Source: three-view drawing plus pictorial views. Frame: mm from the lowest corner of the part. A direction names the side the tool comes from. Give positions to 0.01 mm unless a question says otherwise; leave off trailing zeros. Write each loop counter-clockwise with the first axis right and the second up, starting at its lowest first coordinate (ties: lowest second). Pieces come first, ordered by that corner, then holes.
Q1. Line query: L1, parallel to Y at x = 5.9, z = 7.75; L2, parallel to Y at x = 5, z = 9.75; L3, parallel to Z at x = 1.5, y = 10.25. Output: solid intervals per line, ascending.
Q2. Cut plane D-D on x = 9.25. Return the cut outline in (y, z).
Q3. Cut plane A-A on z = 10. Return the cut outline in (x, y).
Q4. Draft query along X for the marked faces 1, 2 and 3. Return one class per face: pulls with the +X half, pulls with the -X half, needs draft (parallel to the pull), parting line crosses it, or undercut.
Q5. Cut plane B-B on y = 6.25. Return the cut outline in (x, z), plus the area to 3 significant figures.
Q6. Reachability of the marked faces 4 and 5 from +Z, -Z, +X, -X, +Y, -Y: full face, straight path, thin tool, end or side. Return the list, or none.
Q7. Pin query (flat end, axial travel): pin 1 (0.8 mm diameter, centred on x = 5.5, y = 6, fed in from +Z). Return the tip coordinate at first contact, or that it passes through.
Q8. Cut plane C-C on x = 5.9. Return the cut outline in (y, z).
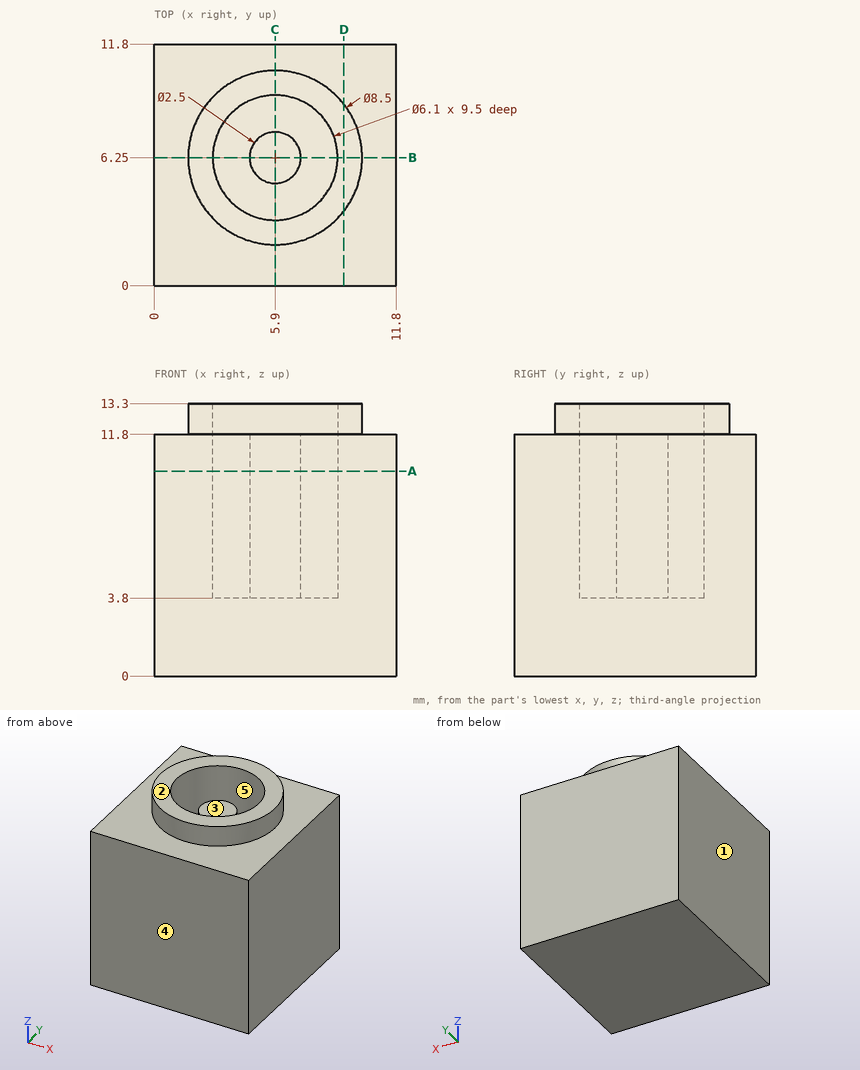
Data:
1. L1: y = 0 to 3.2, 5 to 7.5, 9.3 to 11.8
1. L2: y = 0 to 3.34, 5.38 to 7.12, 9.16 to 11.8
1. L3: z = 0 to 11.8
2. outline: (0, 0) - (11.8, 0) - (11.8, 11.8) - (8.87, 11.8) - (8.87, 13.3) - (3.63, 13.3) - (3.63, 11.8) - (0, 11.8) - close
3. outline: (0, 0) - (11.8, 0) - (11.8, 11.8) - (0, 11.8) - close; circle Ø2.5 at (5.9, 6.25); hole circle Ø6.1 at (5.9, 6.25)
4. face 1: pulls with the -X half
4. face 2: needs draft
4. face 3: undercut
5. outline: (0, 0) - (11.8, 0) - (11.8, 11.8) - (10.15, 11.8) - (10.15, 13.3) - (8.95, 13.3) - (8.95, 3.8) - (7.15, 3.8) - (7.15, 11.8) - (4.65, 11.8) - (4.65, 3.8) - (2.85, 3.8) - (2.85, 13.3) - (1.65, 13.3) - (1.65, 11.8) - (0, 11.8) - close
5. area: 114 mm2
6. face 4: +Z, -Z, +X, -X, -Y
6. face 5: +Z
7. pin 1: stops at z = 11.8
8. outline: (0, 0) - (11.8, 0) - (11.8, 11.8) - (10.5, 11.8) - (10.5, 13.3) - (9.3, 13.3) - (9.3, 3.8) - (7.5, 3.8) - (7.5, 11.8) - (5, 11.8) - (5, 3.8) - (3.2, 3.8) - (3.2, 13.3) - (2, 13.3) - (2, 11.8) - (0, 11.8) - close
